from build123d import *

# Parameters (mm, degrees)
F0_W     = 3
F0_H     = 78
F1_DEPTH = 21
F2_R     = 2
F0_W_2   = 97
F3_DEPTH = 3
F4_W     = 10
F4_H     = 5
F5_DEPTH = 3
F6_R     = 2.5
F7_DEPTH = 10
F4_W_2   = 12.5
F4_H_2   = 6
F8_DEPTH = 3


with BuildPart() as f1:
    # F0 (on Front) → F1 (new body)
    with BuildSketch(Plane.XZ):
        Polygon((-37.858943, 31.427674), (-34.858943, 31.427674), (62.141057, 31.427674), (65.141057, 31.427674), (65.141057, 34.427674), (-37.858943, 34.427674), align=None)
        with Locations((-36.358943, -7.572326)):
            Rectangle(F0_W, F0_H)
        Polygon((62.141057, -46.572326), (-34.858943, -46.572326), (-37.858943, -46.572326), (-37.858943, -49.572326), (65.141057, -49.572326), (65.141057, -46.572326), align=None)
        with Locations((63.641057, -7.572326)):
            Rectangle(F0_W, F0_H)
    extrude(amount=F1_DEPTH)

    # F2
    f2_edges = [f1.edges().sort_by_distance(p)[0] for p in [
        (-37.858943, -10.5, -49.572326),
        (65.141057, -10.5, -49.572326),
        (13.641057, 0, -49.572326),
        (-37.858943, 0, -7.572326),
        (-37.858943, -10.5, 34.427674),
        (13.641057, 0, 34.427674),
        (65.141057, -10.5, 34.427674),
        (65.141057, 0, -7.572326),
    ]]
    fillet(f2_edges, radius=F2_R)

    # F0 (on Front) → F3 (join)
    with BuildSketch(Plane.XZ):
        with Locations((13.641057, -7.572326)):
            Rectangle(F0_W_2, F0_H)
    extrude(amount=F3_DEPTH)

    # F4 (on face) → F5 (cut)
    with BuildSketch(Plane(origin=(0, 0, 31.427674), x_dir=(1, 0, 0), z_dir=(0, 0, -1))):
        with Locations((-9.054972, 5.5)):
            Rectangle(F4_W, F4_H)
    extrude(amount=-F5_DEPTH, mode=Mode.SUBTRACT)

    # F6 (on face) → F7 (join)
    with BuildSketch(Plane.XZ.offset(21)):
        with BuildLine():
            Line((70.641057, 31.426914), (65.141057, 31.426914))
            Line((65.141057, 31.426914), (65.141057, 21.426914))
            Line((65.141057, 21.426914), (70.641057, 21.426914))
            ThreePointArc((70.641057, 21.426914), (75.641057, 26.426914), (70.641057, 31.426914))
        make_face()
        with Locations((70.641057, 26.426914)):
            Circle(F6_R, mode=Mode.SUBTRACT)
        with BuildLine():
            Line((-43.358943, -46.570901), (-37.858943, -46.570901))
            Line((-37.858943, -46.570901), (-37.858943, -36.570901))
            Line((-37.858943, -36.570901), (-43.358943, -36.570901))
            ThreePointArc((-43.358943, -36.570901), (-48.358943, -41.570901), (-43.358943, -46.570901))
        make_face()
        with Locations((-43.358943, -41.570901)):
            Circle(F6_R, mode=Mode.SUBTRACT)
    extrude(amount=-F7_DEPTH)

    # F4 (on face) → F8 (cut)
    with BuildSketch(Plane(origin=(0, 0, 31.427674), x_dir=(1, 0, 0), z_dir=(0, 0, -1))):
        with Locations((21.521203, 6)):
            Rectangle(F4_W_2, F4_H_2)
    extrude(amount=-F8_DEPTH, mode=Mode.SUBTRACT)


solid = f1.part
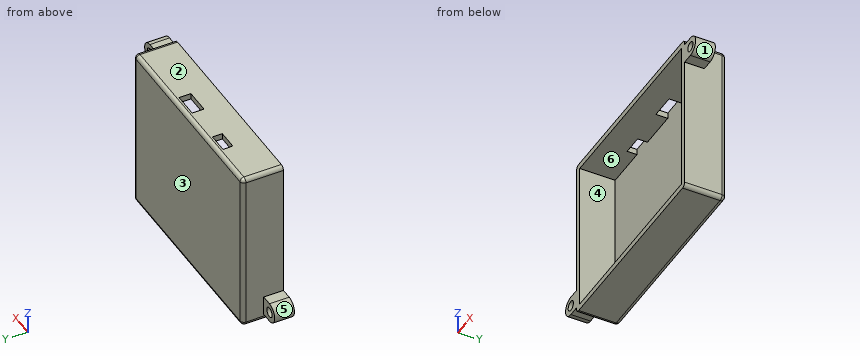
Here's how the part is built. I have some questions about the finished solid (model axes, mm). Face numbers are marked on the shaded views. A direction names the side the tool comes from. Coordinates: 2 decimals unless noted, no trailing zeros. Write each loop counter-clockwise with the first axis right and the second up, starting at its lowest first coordinate (ties: lowest second). Pieces come first, ordered by that corner, then holes.
Item 1: If I drill on line 1 (Z direction, x = 33.5, y = -14); line 2 (Z direction, x = -43, y = -18.75) (3 decimals); line 3 (X direction, y = -14, z = -1), over which ranges is the centre line in solid material (lowest first)?
Item 2: Will these pins go through, and if not, where does the flat tip stop? pin 1 (5 mm diameter, centred on y = -10.5, z = -33, fed in from -X); pin 2 (8 mm diameter, centred on y = -17.5, z = 9, fed in from +X); pin 3 (6.5 mm diameter, centred on x = 70.64, z = 26.43, fed in from +Y).
Item 3: If we mould it in two halves opening along Z, with no side actions, what happens to the marked faces 1, 2, 3 and 4? For each: +Z half, -Z half, draft (parallel to the pull), parting line (faces both ways), or undercut.
Item 4: I want a section at C-C on z = -9. Write out the boundary of the cut face in (x, y).
Item 5: I want a section at B-B on x = -16. Write out the boundary of the cut face in (y, z), and give its area (3 significant figures).
Item 6: I want a section at D-D on y = -13.25. Write out the boundary of the cut face in (x, z).
Item 7: On a 3-axis mill with a long thin cutter (end or side, diameter ignored), from which of +Z, -Z, +X, -X, +Y, -Y can I reach the whole of each face in a straight line? I mean the marked faces 5 and 6. Say none if no direction works.
Item 8: I want a section at A-A on x = 16.5. Write out the boundary of the cut face in (y, z), and give its area (3 significant figures).
Findings below:
1. line 1: z = -49.57 to -46.57, 31.43 to 34.43
1. line 2: z = -46.571 to -44.045, -39.097 to -36.571
1. line 3: x = -37.86 to -34.86, 62.14 to 65.14
2. pin 1: stops at x = -37.86
2. pin 2: stops at x = 65.14
2. pin 3: stops at y = -11
3. face 1: parting line
3. face 2: +Z half
3. face 3: draft
3. face 4: undercut
4. outline: (-37.86, -21) - (-34.86, -21) - (-34.86, -3) - (62.14, -3) - (62.14, -21) - (65.14, -21) - (65.14, -2) arc R2 ccw to (63.14, 0) - (-35.86, 0) arc R2 ccw to (-37.86, -2) - close
5. outline: (-21, -49.57) - (-2, -49.57) arc R2 ccw to (0, -47.57) - (0, 32.43) arc R2 ccw to (-2, 34.43) - (-21, 34.43) - (-21, 31.43) - (-3, 31.43) - (-3, -46.57) - (-21, -46.57) - close
5. area: 358 mm2
6. outline: (-43.36, -46.57) - (-37.86, -46.57) - (-37.86, -47.57) arc R2 ccw to (-35.86, -49.57) - (63.14, -49.57) arc R2 ccw to (65.14, -47.57) - (65.14, 21.43) - (70.64, 21.43) arc R5 ccw to (70.64, 31.43) - (65.14, 31.43) - (65.14, 32.43) arc R2 ccw to (63.14, 34.43) - (-35.86, 34.43) arc R2 ccw to (-37.86, 32.43) - (-37.86, -36.57) - (-43.36, -36.57) arc R5 ccw to start; hole circle Ø5 at (-43.36, -41.57); hole (-34.86, -46.57) - (62.14, -46.57) - (62.14, 31.43) - (-34.86, 31.43) - close; hole circle Ø5 at (70.64, 26.43)
7. face 5: -X, +Y, -Y
7. face 6: -Y
8. outline: (-21, -49.57) - (-2, -49.57) arc R2 ccw to (0, -47.57) - (0, 32.43) arc R2 ccw to (-2, 34.43) - (-3, 34.43) - (-3, -46.57) - (-21, -46.57) - close; (-21, 31.43) - (-9, 31.43) - (-9, 34.43) - (-21, 34.43) - close
8. area: 340 mm2
